```python
from build123d import *

# Parameters (mm, degrees)
SKETCH_1_R          = 2
SKETCH_1_W          = 3
SKETCH_1_H          = 50
SKETCH_1_R_2        = 70
SKETCH_1_R_3        = 20
EXTRUDE_1_DEPTH     = 5
SKETCH_2_R          = 2
CUT_EXTRUDE_1_DEPTH = 697.437362582
SKETCH_3_R          = 2
CUT_EXTRUDE_2_DEPTH = 697.437362582
SKETCH_4_R          = 2
CUT_EXTRUDE_3_DEPTH = 10


with BuildPart() as part:
    # 草图1 → 凸台-拉伸1 (new body)
    # profile 1 of 2: a face of its own
    with BuildSketch(Plane.XY):
        with BuildLine():
            ThreePointArc((-184.975195398, 573.957266214), (-108.724882678, 291.977251427), (-100, 0))
            Line((-100, 0), (-100, -10))
            Line((-100, -10), (-91, -10))
            Line((-91, -10), (-91, 11))
            Line((-91, 11), (-69, 11))
            Line((-69, 11), (-69, -10))
            Line((-69, -10), (100, -10))
            Line((100, -10), (100, 0))
            ThreePointArc((100, 0), (62.740102222, 327.663103245), (-58.911784918, 634.179379428))
            ThreePointArc((-58.911784918, 634.179379428), (-52.264577008, 617.661043914), (-50, 600))
            ThreePointArc((-50, 600), (-106.738470636, 531.267679808), (-184.975195398, 573.957266214))
        make_face()
        with Locations((-50, 0)):
            Circle(SKETCH_1_R, mode=Mode.SUBTRACT)
        Circle(SKETCH_1_R, mode=Mode.SUBTRACT)
        with Locations((50, 0)):
            Circle(SKETCH_1_R, mode=Mode.SUBTRACT)
        with Locations((-91.5, 435)):
            Rectangle(SKETCH_1_W, SKETCH_1_H, mode=Mode.SUBTRACT)
        with Locations((-68.5, 435)):
            Rectangle(SKETCH_1_W, SKETCH_1_H, mode=Mode.SUBTRACT)
    # profile 2 of 2: a face of its own
    with BuildSketch(Plane.XY):
        with Locations((-120, 600)):
            Circle(SKETCH_1_R_2)
        with Locations((-120, 600)):
            Circle(SKETCH_1_R_3, mode=Mode.SUBTRACT)
    extrude(amount=EXTRUDE_1_DEPTH)

    # 草图2 → 切除-拉伸1 (cut, through all)
    with BuildSketch(Plane(origin=(0, 0, 0), x_dir=(-1, 0, 0), z_dir=(0, 0, -1))):
        with Locations((80, 386.410161514)):
            Circle(SKETCH_2_R)
        with Locations((80, 371.410161514)):
            Circle(SKETCH_2_R)
        with Locations((80, 356.410161514)):
            Circle(SKETCH_2_R)
        with Locations((56.339745962, 352.749907476)):
            Circle(SKETCH_2_R)
        with Locations((46.339745962, 335.4293994)):
            Circle(SKETCH_2_R)
        with Locations((26.339745962, 300.788383249)):
            Circle(SKETCH_2_R)
        with Locations((6.339745962, 266.147367097)):
            Circle(SKETCH_2_R)
        with Locations((-13.660254038, 231.506350946)):
            Circle(SKETCH_2_R)
        with Locations((80, 76.410161514)):
            Circle(SKETCH_2_R)
        with Locations((80, 116.410161514)):
            Circle(SKETCH_2_R)
        with Locations((80, 236.410161514)):
            Circle(SKETCH_2_R)
        with Locations((80, 276.410161514)):
            Circle(SKETCH_2_R)
        with Locations((80, 316.410161514)):
            Circle(SKETCH_2_R)
    extrude(amount=-CUT_EXTRUDE_1_DEPTH, mode=Mode.SUBTRACT)

    # 草图3 → 切除-拉伸2 (cut, through all)
    with BuildSketch(Plane.XY.offset(5)):
        with Locations((-165, 625)):
            Circle(SKETCH_3_R)
        with Locations((-75, 625)):
            Circle(SKETCH_3_R)
        with Locations((-75, 575)):
            Circle(SKETCH_3_R)
        with Locations((-165, 575)):
            Circle(SKETCH_3_R)
        with Locations((-168.657553327, 583.19397417)):
            Circle(SKETCH_3_R)
        with Locations((-159.975144444, 632.43436182)):
            Circle(SKETCH_3_R)
        with Locations((-71.342446673, 616.80602583)):
            Circle(SKETCH_3_R)
        with Locations((-80.024855556, 567.56563818)):
            Circle(SKETCH_3_R)
        with Locations((-86.264335648, 638.883221969)):
            Circle(SKETCH_3_R)
        with Locations((-69.163328481, 591.89859093)):
            Circle(SKETCH_3_R)
        with Locations((-153.735664352, 561.116778031)):
            Circle(SKETCH_3_R)
        with Locations((-170.836671519, 608.10140907)):
            Circle(SKETCH_3_R)
        with Locations((-101.597690302, 648.076553514)):
            Circle(SKETCH_3_R)
        with Locations((-69.458309817, 609.774331358)):
            Circle(SKETCH_3_R)
        with Locations((-138.402309698, 551.923446486)):
            Circle(SKETCH_3_R)
        with Locations((-170.541690183, 590.225668642)):
            Circle(SKETCH_3_R)
    extrude(amount=-CUT_EXTRUDE_2_DEPTH, mode=Mode.SUBTRACT)


with BuildPart() as body_2:
    # Split Bodies 1: the piece on the far side of the plane
    add(part.part)
    split(bisect_by=Plane(origin=(0, 325, 0), x_dir=(0, 0, -1), z_dir=(0, -1, 0)), keep=Keep.BOTTOM)

    # 草图4 → 切除-拉伸3 (cut)
    with BuildSketch(Plane.XY.offset(5)):
        with Locations((-21.595687559, 455)):
            Circle(SKETCH_4_R)
        with BuildLine():
            Line((-11.595687559, 325), (-11.595687559, 540.604962521))
            ThreePointArc((-11.595687559, 540.604962521), (30.836385122, 434.518144234), (63.404312441, 325))
            Line((63.404312441, 325), (-11.595687559, 325))
        make_face()
    extrude(amount=-CUT_EXTRUDE_3_DEPTH, mode=Mode.SUBTRACT)


with BuildPart() as part_1:
    add(part.part)

    # Split Bodies 1
    split(bisect_by=Plane(origin=(0, 325, 0), x_dir=(0, 0, -1), z_dir=(0, -1, 0)), keep=Keep.TOP)


solid = body_2.part
```
Could you check a few things on this model? Use its own coordinates, in mm. Give positions to 0.01 mm unless a question says otherwise; leave off trailing zeros. Loops run counter-clockwise (first coordinate to the right, second up) from the corner with the lowest first, then second, coordinate; pieces in that order, holes last. Notation, with made-up numbers: (-37.75, 52.5) - (-13.75, 52.5) arc R12 ccw to (-13.75, 74.5) - close; hole circle Ø11 at (-7.5, 27). An arc over 180 degrees is marked (long way). Use one line per item in the form item = value.
1. I want a section at D-D (z = 3). Give the number of separate pieces and of enclosed holes in the cut face, and give its area (3 significant figures).
Response values:
separate_pieces = 1
enclosed_holes = 25
area = 42,900 mm²
2. I want a section at C-C (y = 600). Please give me the cut outline in (x, z), and give its area (3 significant figures).
Response values:
outline = (-190, 0) - (-140, 0) - (-140, 5) - (-190, 5) - close; (-100, 0) - (-40.48, 0) - (-40.48, 5) - (-100, 5) - close
area = 548 mm²
3. I want a section at A-A (y = 439.5). Please give me the cut outline in (x, z), and give its area (3 significant figures).
Response values:
outline = (-139.76, 0) - (-93, 0) - (-93, 5) - (-139.76, 5) - close; (-90, 0) - (-70, 0) - (-70, 5) - (-90, 5) - close; (-67, 0) - (-11.6, 0) - (-11.6, 5) - (-67, 5) - close
area = 611 mm²
4. I want a section at B-B (x = -120). Please give me the cut outline in (y, z), and give its area (3 significant figures).
Response values:
outline = (356.44, 0) - (580, 0) - (580, 5) - (356.44, 5) - close; (620, 0) - (670, 0) - (670, 5) - (620, 5) - close
area = 1,370 mm²
5. I'm going to push flat-ended pins straight in: pin 1 Ø3.5 at (x, y) = (-69.46, 609.77) entering from -Z (3 decimals); pin 2 Ø3 at (x, z) = (-149, 1) entering from +Y; pin 3 Ø1 at (x, z) = (-79, 3) entering from +Y. Where does each tip first touch, or does it pass through?
Response values:
pin_1 = through
pin_2 = 664.37
pin_3 = 657.09
6. I need wall thicknesses on probe 1 along X at (y, z) = (625, 1.25); probe 2 along Y at (x, z) = (-75, 1.2); probe 3 along Y at (x, z) = (-80, 2.5). Which ranges of each line are inside material? Lowest first, please.
Response values:
probe_1 = -185.38 to -167, -163 to -77, -73 to -53.83
probe_2 = 325 to 573, 577 to 623, 627 to 653.62
probe_3 = 325 to 354.41, 358.41 to 369.41, 373.41 to 384.41, 388.41 to 565.57, 569.57 to 657.45
7. Thinking about a two-plate mould opening in X: for faces 1 (the face through (-143.557, 453.065, 2.465)), 2 (the face through (-124.336, 580.476, 2.465)), 3 (the face through (-82, 500, 5)), which applies, released by +X, released by -X, zero draft, split by the parting line, or undercut?
Response values:
face_1 = released by -X
face_2 = undercut
face_3 = zero draft
